Source: CAD feature listing. Evaluate the final solid. Frame: model axes, mm. Round coordinates to 2 decimals unless told otherwise and drop trailing zeros. Write each loop counter-clockwise with the first axis right and the second up, starting at its lowest first coordinate (ties: lowest second). Pieces come first, ordered by that corner, then holes. Notation, with made-up numbers: M 1.5,52 L 12.5,52 A27 cw 12.5,72 Z; hole C 40.25,84 d7. An arc over 180 degrees is marked long. Use a Markdown table: item, result.
```python
from build123d import *

# Parameters (mm, degrees)
F0_R     = 10
F0_R_2   = 4.25
F1_DEPTH = 30
F2_R     = 23.5
F2_R_2   = 19
F3_DEPTH = 12


with BuildPart() as f1:
    # F0 (on Front) → F1 (new body)
    with BuildSketch(Plane.XZ):
        Circle(F0_R)
        Circle(F0_R_2, mode=Mode.SUBTRACT)
    extrude(amount=F1_DEPTH)

    # F2 (on Right) → F3 (join)
    with BuildSketch(Plane.YZ):
        with Locations((-49, 0)):
            Circle(F2_R)
        with Locations((-49, 0)):
            Circle(F2_R_2, mode=Mode.SUBTRACT)
    extrude(amount=F3_DEPTH)

    # F4: F1 across plane


with BuildPart() as f1_1:
    add(f1.part)
    add(f1.part.mirror(Plane.YZ))


solid = f1_1.part
```
Q1. Section D-D on z = 5. Return loops of the section in (x, y).
Results are:
| item | result |
|---|---|
| outline | M -12,-71.96 L 12,-71.96 L 12,-67.33 L -12,-67.33 Z; M -12,-30.67 L 12,-30.67 L 12,-26.04 L 8.66,-26.04 L 8.66,0 L -8.66,0 L -8.66,-26.04 L -12,-26.04 Z |
Q2. Section B-B on z = -8.5. Return loops of the section in (x, y).
Results are:
| item | result |
|---|---|
| outline | M -12,-70.91 L 12,-70.91 L 12,-65.99 L -12,-65.99 Z; M -12,-32.01 L 12,-32.01 L 12,-27.09 L 5.27,-27.09 L 5.27,0 L -5.27,0 L -5.27,-27.09 L -12,-27.09 Z |
Q3. Section A-A on y = -49. Return loops of the section in (x, z), plus the area to 3 significant figures.
Results are:
| item | result |
|---|---|
| outline | M -12,-23.5 L 12,-23.5 L 12,-19 L -12,-19 Z; M -12,19 L 12,19 L 12,23.5 L -12,23.5 Z |
| area | 216 mm^2 |
Q4. First-contact query: pin 1 Ø5 at (x, y) = (6.5, -15.5) entering from +Z; pin 2 Ø1 at (x, y) = (8.5, -22.5) entering from -Z; pin 3 Ø1 at (y, z) = (-14.5, 7) entering from -X. Flat tips, straight axial feed; report the tip coordinate or a pass-through.
Results are:
| item | result |
|---|---|
| pin 1 | z = 9.17 |
| pin 2 | z = -6 |
| pin 3 | x = -7.6 |
Q5. Line query: L1, parallel to Z at x = 4.75, y = -49; L2, parallel to Z at x = 0, y = -8. Output: solid intervals per line, ascending.
Results are:
| item | result |
|---|---|
| L1 | -23.5 to -19, 19 to 23.5 |
| L2 | -10 to -4.25, 4.25 to 10 |
Q6. Section C-C on x = 2.25. Return loops of the section in (y, z), plus the area to 3 significant figures.
Results are:
| item | result |
|---|---|
| outline | M -27.62,-9.74 L 0,-9.74 L 0,-3.61 L -25.78,-3.61 A23.5 ccw -25.78,3.61 L 0,3.61 L 0,9.74 L -27.62,9.74 A23.5 ccw long Z; hole C -49,0 d38 |
| area | 927 mm^2 |
Q7. Mould query, pull axis Z, two halves, no side actions, for faces 1 (the cylindrical face through (-10, -14, 0)), 2 (the flat face through (4, 0, -2)), 3 (the cylindrical face through (2.285, -12.763, 3.584)). Classes: +Z half, -Z half, draft (parallel to the pull), parting line (faces both ways), or undercut.
Results are:
| item | result |
|---|---|
| face 1 | parting line |
| face 2 | draft |
| face 3 | undercut |
